Input: part model. Units: mm. Frame: model coordinates. Give positions to 0.01 mm unless a question says otherwise; leave off trailing zeros. Order: outer loops, then holes, each group sorted by start corner. A loop starts at its lowest first (then second) coordinate and runs counter-clockwise, first axis right, second up. Notation, with made-up numbers: M -25.75,57.5 L -13.75,57.5 A18 cw -13.75,64.5 Z; hole C -32,-18 d3. An arc over 180 degrees is marked long. Use a Markdown table: item, result.
from build123d import *

# Parameters (mm, degrees)
ESQUISSE1_R                 = 7.5
BOSS_EXTRU_1_DEPTH          = 60
ESQUISSE6_W                 = 6
ESQUISSE6_H                 = 6
BOSS_EXTRU_2_DEPTH          = 1
ENL_V_MAT_EXTRU_2_OUTLINE_W = 2.5
ENL_V_MAT_EXTRU_2_OUTLINE_H = 15.000451996


# Read off the part's stored shape, not the designer's step: Enlèv. mat.-Extru.2
with BuildPart() as part:
    # Esquisse1 → Boss.-Extru.1 (new body)
    with BuildSketch(Plane.XY):
        Circle(ESQUISSE1_R)
    boss_extru_1 = extrude(amount=BOSS_EXTRU_1_DEPTH)

    # Esquisse6 → Boss.-Extru.2 (add)
    with BuildSketch(Plane(origin=(0, 0, 0), x_dir=(-1, 0, 0), z_dir=(0, 0, -1))):
        Rectangle(ESQUISSE6_W, ESQUISSE6_H)
    boss_extru_2 = extrude(amount=BOSS_EXTRU_2_DEPTH)

    # Enlèv. mat.-Extru.2 outline → Enlèv. mat.-Extru.2 (revolve, cut)
    with BuildSketch(Plane(origin=(-0.054510378, 0, 5), x_dir=(1, 0, 0), z_dir=(0, 0, 1))):
        with Locations((1.25, 0)):
            Rectangle(ENL_V_MAT_EXTRU_2_OUTLINE_W, ENL_V_MAT_EXTRU_2_OUTLINE_H)
    enl_v_mat_extru_2 = revolve(axis=Axis((-0.054510378, 0, 5), (0, 1, 0)), mode=Mode.SUBTRACT)

    # Symétrie4: Boss.-Extru.1, Boss.-Extru.2, Enlèv. mat.-Extru.2 across plane
    add(boss_extru_1.mirror(Plane.XY.offset(60)))
    add(boss_extru_2.mirror(Plane.XY.offset(60)))
    add(enl_v_mat_extru_2.mirror(Plane.XY.offset(60)), mode=Mode.SUBTRACT)


solid = part.part
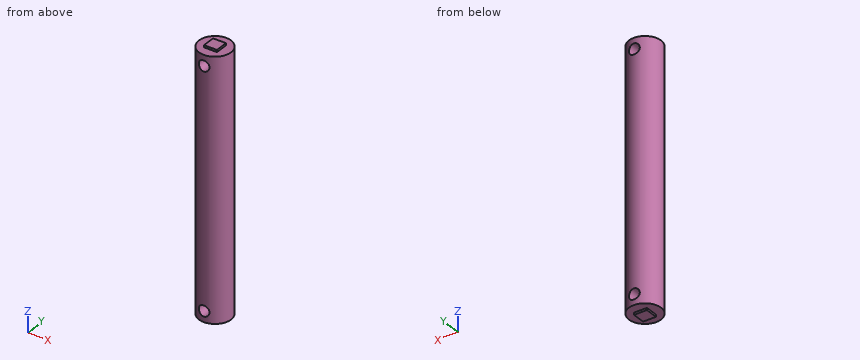
1) Cut plane B-B on x = 0. Return loops of the section in (y, z), and give its area (3 significant figures).
Response values:
| item | result |
|---|---|
| outline | M -7.5,0 L -3,0 L -3,-1 L 3,-1 L 3,0 L 7.5,0 L 7.5,2.5 L -7.5,2.5 Z; M -7.5,7.5 L 7.5,7.5 L 7.5,112.5 L -7.5,112.5 Z; M -7.5,117.5 L 7.5,117.5 L 7.5,120 L 3,120 L 3,121 L -3,121 L -3,120 L -7.5,120 Z |
| area | 1,660 mm² |
2) Cut plane D-D on y = 4.5. Return loops of the section in (x, z), and give its area (3 significant figures).
Response values:
| item | result |
|---|---|
| outline | M -6,0 L 6,0 L 6,120 L -6,120 Z; hole C -0.05,5 d5; hole C -0.05,115 d5 |
| area | 1,400 mm² |
3) Material intervals for line 1 (Z direction, x = -0.25, y = -0.25); line 2 (Z direction, x = -1, y = -6); line 3 (X direction, y = 0.25, z = 16), sorted ascending. Write a range as from..to.
Response values:
| item | result |
|---|---|
| line 1 | z = -1..2.51, 7.49..112.51, 117.49..121 |
| line 2 | z = 0..2.69, 7.31..112.69, 117.31..120 |
| line 3 | x = -7.5..7.5 |
4) Cut plane A-A on y = 0. Return loops of the section in (x, z), and give its area (3 significant figures).
Response values:
| item | result |
|---|---|
| outline | M -7.5,0 L -3,0 L -3,-1 L 3,-1 L 3,0 L 7.5,0 L 7.5,120 L 3,120 L 3,121 L -3,121 L -3,120 L -7.5,120 Z; hole C -0.05,5 d5; hole C -0.05,115 d5 |
| area | 1,770 mm² |
5) Cut plane C-C on z = 38. Return loops of the section in (x, y), and give its area (3 significant figures).
Response values:
| item | result |
|---|---|
| outline | C 0,0 d15 |
| area | 177 mm² |
6) First-contact query: pin 1 Ø4.5 at (x, z) = (-0.05, 115) entering from +Y; pin 2 Ø0.8 at (x, z) = (0, 120.5) entering from +Y; pin 3 Ø0.8 at (y, z) = (1, -0.5) entering from -X; pin 4 Ø1 at (x, z) = (-1, 84) entering from +Y. Flat tips, straight axial feed; report the tip coordinate or a pass-through.
Response values:
| item | result |
|---|---|
| pin 1 | passes through |
| pin 2 | stops at y = 3 |
| pin 3 | stops at x = -3 |
| pin 4 | stops at y = 7.48 |
